Design review of the part built by this model. Coordinates are the model's own, in mm. A direction names the side the tool comes from. Round coordinates to 2 decimals unless told otherwise and drop trailing zeros. Write each loop counter-clockwise with the first axis right and the second up, starting at its lowest first coordinate (ties: lowest second). Pieces come first, ordered by that corner, then holes. Notation, with made-up numbers: (-21, 86.25) - (2, 86.25) arc R11 cw to (2, 100.25) - close; hole circle Ø9 at (46.5, -14.5). An arc over 180 degrees is marked (long way). Use one line per item in the form item = value.
Autodesk Inventor part; units mm, degrees
ref_plane "YZ Plane" through (0, 0, 0) normal (1, 0, 0) x (0, 1, 0)
ref_plane "XZ Plane" through (0, 0, 0) normal (0, 1, 0) x (-1, 0, 0)
ref_plane "XY Plane" through (0, 0, 0) normal (0, 0, 1) x (1, 0, 0)
sketch "Sketch1" plane through (0, 0, 0) normal (0, 0, 1) x (1, 0, 0)
  line L0 (0, 0) -> (3.175, 0)
  line L1 (3.175, 0) -> (3.175, 50.8)
  line L2 (3.175, 50.8) -> (0, 50.8)
  line L3 (0, 50.8) -> (0, 0)
  line L4 (0, 0) -> (50.8, 0)
  line L5 (50.8, 0) -> (50.8, 3.175)
  line L6 (50.8, 3.175) -> (0, 3.175)
  line L7 (0, 3.175) -> (0, 0)
  dimension "d0" = 3.175
  dimension "d1" = 50.8
  dimension "d2" = 50.8
  dimension "d3" = 3.175
extrude "Extrusion1" add sketch "Sketch1" along normal blind 25.4
sketch "Sketch2" plane through (3.175, 3.175, 0) normal (1, 0, 0) x (0, 0, -1)
  line L0 (0, 47.625) -> (-25.4, 47.625) construction
  line L1 (-12.7, 47.625) -> (-12.7, 34.925) construction
  line L2 (-12.7, 34.925) -> (-12.7, 9.525) construction
  circle A0 centre (-12.7, 34.925) radius 2.5797
  circle A1 centre (-12.7, 9.525) radius 2.5797
  point P0 (0, -3.175)
  dimension "d6" = 12.7
  dimension "d7" = 25.4
  dimension "d8" = 5.1594
extrude "Extrusion2" cut sketch "Sketch2" against normal blind 25.4
properties part number "2x2 L"
Q1. Draft analysis for pull direction Z (two halves, no side actions). For faces 3 (the cylindrical face through (1.61, 35.81, 11.51)), 4 (the flat face through (3, 14, 25.4)), 5 (the flat face through (25, 0, 13)), state which applies: released by +Z, released by -Z, zero draft, split by the parting line, or undercut.
Calculated:
face_3 = undercut
face_4 = released by +Z
face_5 = zero draft
Q2. Machinability: for faces 1 (the flat face through (27, 3.175, 13)), 2 (the flat face through (2, 50.8, 13)), which of the approach directions +Z, -Z, +X, -X, +Y, -Y give a long, thin tool a straight path to every point of the face, cutting with its end or side? Answer none if there is none.
Calculated:
face_1 = +Z, -Z, +X, +Y
face_2 = +Z, -Z, +X, -X, +Y
Q3. We need section D-D on x = 9. Write out the cut boundary in (y, z) (3 decimals).
Calculated:
outline = (0, 0) - (3.175, 0) - (3.175, 25.4) - (0, 25.4) - close
Q4. For P1, Ø12, axis at x = 33, z = 21.5, coming from the +Y side (3 decimals); P2, Ø2, axis at y = 17, z = 5, coming from the +X side (3 decimals), all flat-tipped, find the tip position at first contact; note any pin that passes through.
Calculated:
P1 = 3.175
P2 = 3.175
Q5. We need section B-B on z = 12.7. Write out the cut boundary in (x, y) (3 decimals), then the cut area to 3 significant figures.
Calculated:
outline = (0, 0) - (50.8, 0) - (50.8, 3.175) - (3.175, 3.175) - (3.175, 10.12) - (0, 10.12) - close; (0, 15.28) - (3.175, 15.28) - (3.175, 35.52) - (0, 35.52) - close; (0, 40.68) - (3.175, 40.68) - (3.175, 50.8) - (0, 50.8) - close
area = 280 mm2
Q6. We need section C-C on z = 19.75. Write out the cut boundary in (x, y) (3 decimals), then the cut area to 4 significant figures.
Calculated:
outline = (0, 0) - (50.8, 0) - (50.8, 3.175) - (3.175, 3.175) - (3.175, 50.8) - (0, 50.8) - close
area = 312.5 mm2
Q7. We need section A-A on y = 12.7. Write out the cut boundary in (x, z) (3 decimals).
Calculated:
outline = (0, 0) - (3.175, 0) - (3.175, 10.12) - (0, 10.12) - close; (0, 15.28) - (3.175, 15.28) - (3.175, 25.4) - (0, 25.4) - close
Q8. To check wall thickness, follow line 1 along Y through (x, z) = (2.2, 12.7); line 2 along Z through (x, y) = (1, 38); line 3 along X through (y, z) = (42, 21.75) (3 decimals). State the ranges of each line that lie inside material, in increasing order. Write a range as from..to.
Calculated:
line_1 = 0..10.12, 15.28..35.52, 40.68..50.8
line_2 = 0..10.12, 15.28..25.4
line_3 = 0..3.175
